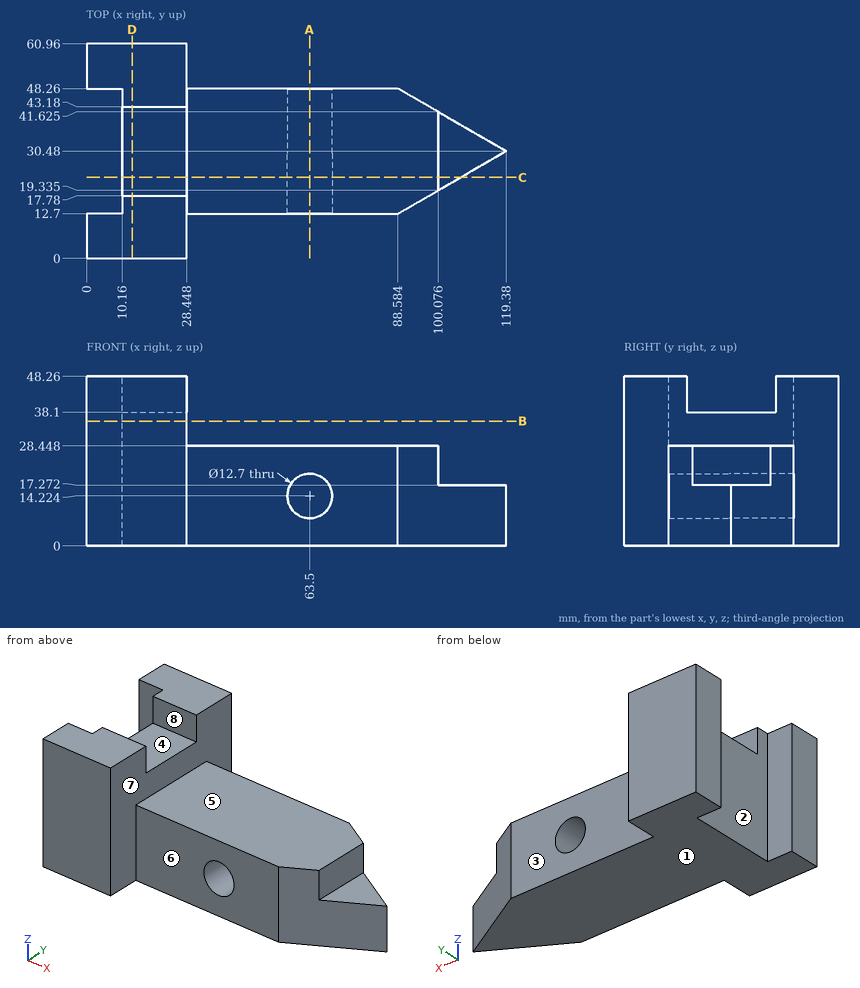
Input: dimensioned drawing with shaded views. Units: mm. Origin: part minimum x, y, z. A direction names the side the tool comes from. Give positions to 0.01 mm unless a question says otherwise; leave off trailing zeros. Write each loop counter-clockwise with the first axis right and the second up, starting at its lowest first coordinate (ties: lowest second). Pieces come first, ordered by that corner, then holes.
Q1. First-contact query: P1, Ø21, axis at x = 108, y = 25.5, coming from the +Z side; P2, Ø16.5, axis at x = 63.5, z = 14.224, coming from the +Y side; P3, Ø2, axis at y = 15.5, z = 42.5, coming from the +X side. Flat tips, straight axial feed; report the tip coordinate or a pass-through.
Q2. Section A-A, the plane x = 63.5. Output: boundary loops of the cut face in (y, z).
Q3. Pull-direction query (Y, two-part tool) for the marked faces 6, 7 and 8; classes: pulls with the +Y half, pulls with the -Y half, needs draft (parallel to the pull), parting line crosses it, or undercut.
Q4. Material intervals for probe 1 along Z at (x, y) = (63.5, 20.75); probe 2 along Y at (x, z) = (27, 40); probe 3 along Z at (x, y) = (13, 42), sorted ascending.
Q5. Set-up query: the marked faces 1, 2, 3, 4 and 5. Return all of +Z, -Z, +X, -X, +Y, -Y with unobstructed straight access to the full face (end or side cutting, diameter ignored); none if empty.
Q6. Section C-C, the plane y = 23. Output: boundary loops of the cut face in (x, z).
Q7. Section D-D, the plane x = 13. Output: boundary loops of the cut face in (y, z).
Q8. Section B-B, the plane z = 35.5. Output: boundary loops of the cut face in (x, y).
Filled in:
1. P1: stops at z = 28.45
1. P2: stops at y = 48.26
1. P3: stops at x = 28.45
2. outline: (12.7, 0) - (48.26, 0) - (48.26, 7.87) - (12.7, 7.87) - close; (12.7, 20.57) - (48.26, 20.57) - (48.26, 28.45) - (12.7, 28.45) - close
3. face 6: pulls with the -Y half
3. face 7: needs draft
3. face 8: undercut
4. probe 1: z = 0 to 7.87, 20.57 to 28.45
4. probe 2: y = 0 to 17.78, 43.18 to 60.96
4. probe 3: z = 0 to 38.1
5. face 1: -Z, +X, -X, +Y, -Y
5. face 2: +Z, -Z, -X
5. face 3: +Z, -Z, +X, +Y
5. face 4: +Z, +X, -X
5. face 5: +Z, +X, +Y, -Y
6. outline: (10.16, 0) - (106.42, 0) - (106.42, 17.27) - (100.08, 17.27) - (100.08, 28.45) - (28.45, 28.45) - (28.45, 38.1) - (10.16, 38.1) - close; hole circle Ø12.7 at (63.5, 14.22)
7. outline: (0, 0) - (60.96, 0) - (60.96, 48.26) - (43.18, 48.26) - (43.18, 38.1) - (17.78, 38.1) - (17.78, 48.26) - (0, 48.26) - close
8. outline: (0, 0) - (28.45, 0) - (28.45, 60.96) - (0, 60.96) - (0, 48.26) - (10.16, 48.26) - (10.16, 12.7) - (0, 12.7) - close
